Geometry: see drawing. Coordinates: mm, zero at the bounding-box minimum. Give positions to 0.01 mm unless a question says otherwise; leave off trailing zeros. Loops run counter-clockwise (first coordinate to the right, second up) from the corner with the lowest first, then second, coordinate; pieces in that order, holes last. Notation, with made-up numbers: M 24.25,-19 L 32.25,-19 A27 ccw 32.25,16 Z; hole C -31,87 d2. An arc over 180 degrees is marked long. Return JSON: item names as keys, results as strings. Group by question number.
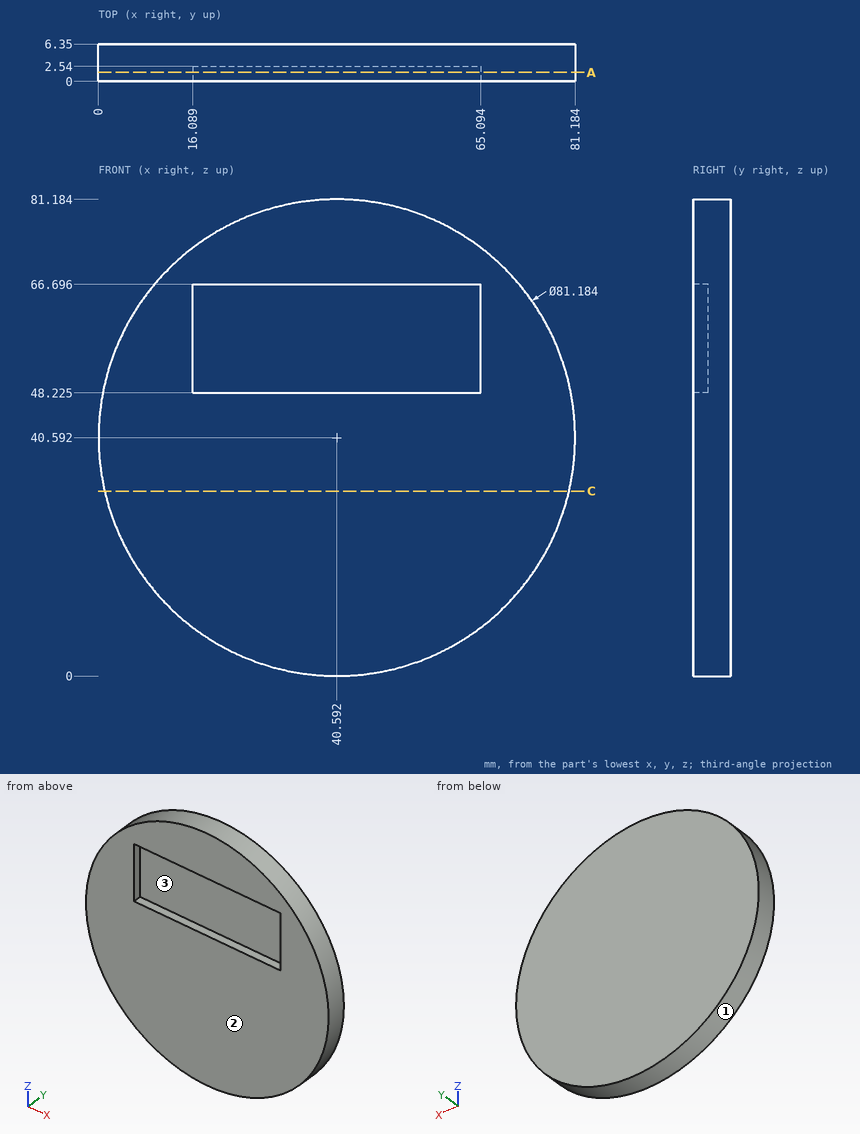
Item 1: Section A-A, the plane y = 1.5. Return loops of the section in (x, z) (1 decimal), then the cut area to 3 significant figures.
Item 2: First-contact query: pin 1 Ø3 at (y, z) = (2.5, 58.5) entering from +X; pin 2 Ø1.3 at (x, y) = (49.5, 1) entering from -Z; pin 3 Ø1.5 at (x, y) = (9, 1) entering from -Z. Flat tips, straight axial feed; report the tip coordinate or a pass-through.
Item 3: Material intervals for line 1 (Z direction, x = 24.5, y = 0.75) (1 decimal); line 2 (Z direction, x = 58.5, y = 1.75) (1 decimal); line 3 (X direction, y = 6, z = 41.5), sorted ascending. Write a range as from..to.
Item 4: Section C-C, the plane z = 31.5. Return loops of the section in (x, y).
Item 5: Pull-direction query (X, two-part tool) for the marked faces 1, 2 and 3; classes: pulls with the +X half, pulls with the -X half, needs draft (parallel to the pull), parting line crosses it, or undercut.
Answer below:
{
 "1": {"outline": "C 40.6,40.6 d81.2; hole M 16.1,48.2 L 65.1,48.2 L 65.1,66.7 L 16.1,66.7 Z", "area": "4,270 mm^2"},
 "2": {"pin 1": "x = 77.72", "pin 2": "z = 0.85", "pin 3": "z = 14.2"},
 "3": {"line 1": "3.3..48.2, 66.7..77.9", "line 2": "4.2..48.2, 66.7..77", "line 3": "0.01..81.17"},
 "4": {"outline": "M 1.03,0 L 80.15,0 L 80.15,6.35 L 1.03,6.35 Z"},
 "5": {"face 1": "parting line crosses it", "face 2": "needs draft", "face 3": "undercut"}
}
